Read the model definition and answer for the solid it produces. Units are mm, in the model's axes. Face numbers are marked on the shaded views. A direction names the side the tool comes from. Coordinates: 2 decimals unless noted, no trailing zeros. Order: outer loops, then holes, each group sorted by start corner. A loop starts at its lowest first (then second) coordinate and runs counter-clockwise, first axis right, second up. Notation, with made-up numbers: (73, 30.5) - (86, 30.5) arc R34 cw to (86, 63.5) - close; hole circle Ø4 at (77.5, -19.75). An arc over 180 degrees is marked (long way). Answer as a JSON object with one key per item and string values. Group by question number.
from build123d import *

# Parameters (mm, degrees)
F0_R     = 9.525
F1_DEPTH = 25.4
F2_R     = 6.35
F3_DEPTH = 19.05
F4_W     = 76.2
F4_H     = 3.175
F5_DEPTH = 304.8


with BuildPart() as f1:
    # F0 (on Front) → F1 (new body)
    with BuildSketch(Plane.XZ):
        Circle(F0_R)
    extrude(amount=-F1_DEPTH)

    # F2 (on face) → F3 (cut)
    with BuildSketch(Plane(origin=(0, 25.4, 0), x_dir=(-1, 0, 0), z_dir=(0, 1, 0))):
        Circle(F2_R)
    extrude(amount=-F3_DEPTH, mode=Mode.SUBTRACT)

    # F4 (on Front) → F5 (join)
    with BuildSketch(Plane.XZ):
        Rectangle(F4_W, F4_H)
    extrude(amount=F5_DEPTH)


solid = f1.part
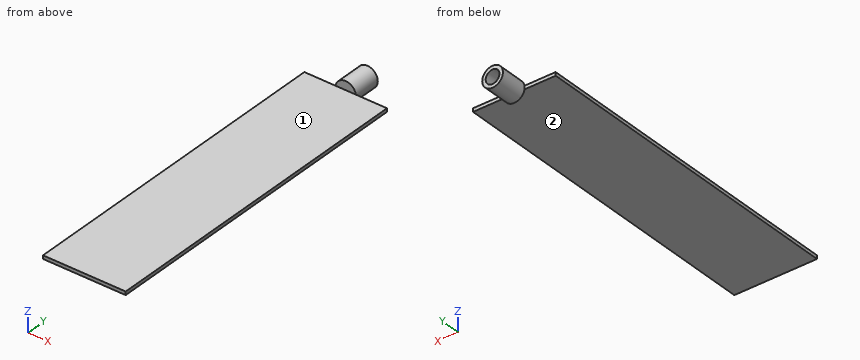
1. A cutting plane is placed at C-C on x = -25.5. Write down the section's boundary in (y, z), and give its area (3 significant figures).
2. Straight lines are drawn through the part: L1, parallel to Z at x = 0, y = 11 (3 decimals); L2, parallel to Y at x = -3, z = 6; L3, parallel to Y at x = 3, z = 4.5. For each, find the intervals that lie inside material, in ascending order.
3. Given pin 1 (23 mm diameter, centred on x = -1, y = -169, fed in from -Z); pin 2 (1.6 mm diameter, centred on x = 18.5, z = 0, fed in from +Y); pin 3 (8 mm diameter, centred on x = -12.5, y = -231.5, fed in from +Z), each flat-ended and moving along its own axis, determine where each tip first touches the part or whether it passes through.
4. A cutting plane is placed at B-B on y = -203.5. Write down the section's boundary in (x, z), and give its area (3 significant figures).
5. For the marked faces 1 and 2, determine the directions among +Z, -Z, +X, -X, +Y, -Y from which every point of the face is accessible in a straight line to the end or side of a thin tool.
Derived:
{
 "1": {"outline": "(-304.8, -1.59) - (0, -1.59) - (0, 1.59) - (-304.8, 1.59) - close", "area": "968 mm2"},
 "2": {"L1": "z = -9.525 to -6.35, 6.35 to 9.525", "L2": "y = 0 to 25.4", "L3": "y = 0 to 6.35"},
 "3": {"pin 1": "stops at z = -1.59", "pin 2": "stops at y = 0", "pin 3": "stops at z = 1.59"},
 "4": {"outline": "(-38.1, -1.59) - (38.1, -1.59) - (38.1, 1.59) - (-38.1, 1.59) - close", "area": "242 mm2"},
 "5": {"face 1": "+Z, +X, -X, -Y", "face 2": "-Z, +X, -X, -Y"}
}
